The drawing under review shows one solid part. Ordinate dimensions are in mm from its lowest x, y, z. Coordinates: 2 decimals unless noted, no trailing zeros. Order: outer loops, then holes, each group sorted by start corner. A loop starts at its lowest first (then second) coordinate and runs counter-clockwise, first axis right, second up.
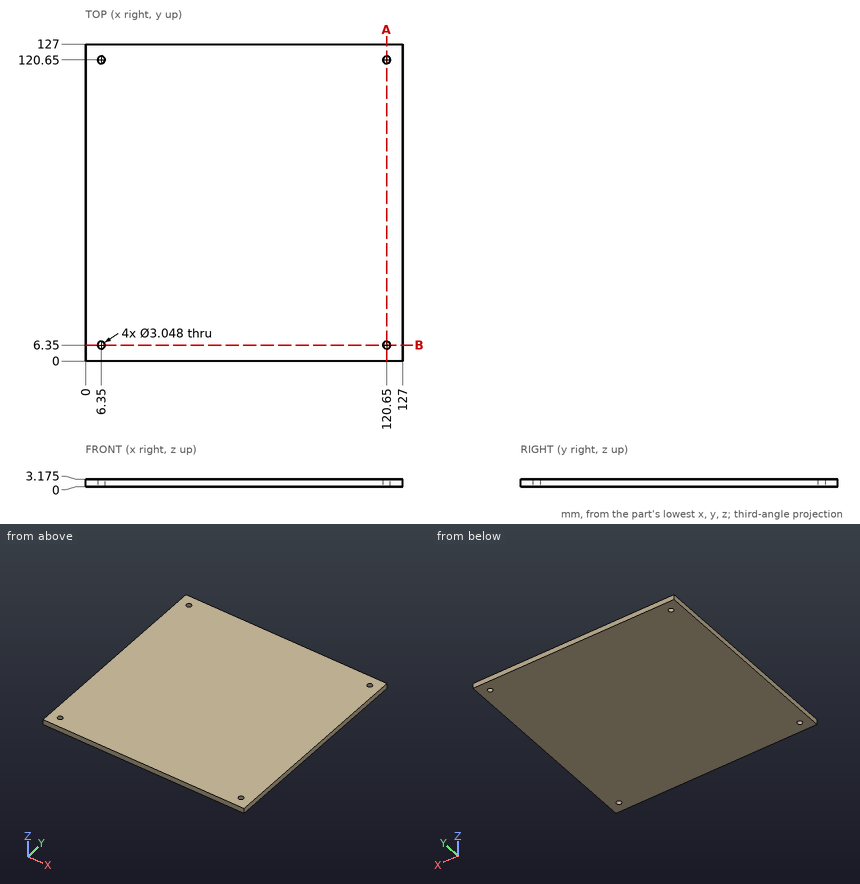
(1) For pin 1 Ø2.5 at (x, y) = (120.65, 6.35) entering from +Z, flat-tipped, find the tip position at first contact; note if it passes through.
A:
pin 1: passes through
(2) We need section A-A, the plane x = 120.65. Write out the cut boundary in (y, z) (3 decimals).
A:
outline: (0, 0) - (4.826, 0) - (4.826, 3.175) - (0, 3.175) - close; (7.874, 0) - (119.126, 0) - (119.126, 3.175) - (7.874, 3.175) - close; (122.174, 0) - (127, 0) - (127, 3.175) - (122.174, 3.175) - close
(3) Wall thickness on probe 1 along Y at (x, z) = (120.65, 2.35): over which ranges is the line inside the solid? List them lowest first.
A:
probe 1: y = 0 to 4.83, 7.87 to 119.13, 122.17 to 127
